from build123d import *

# Parameters (mm, degrees)
SKETCH1_W           = 6.5
SKETCH1_H           = 6
BOSS_EXTRUDE1_DEPTH = 1.75
SKETCH2_W           = 6.52
SKETCH2_H           = 6.02
SKETCH2_R           = 1.505
BOSS_EXTRUDE2_DEPTH = 0.25
SKETCH3_R           = 1.5
BOSS_EXTRUDE3_DEPTH = 1.2
FILLET1_R           = 0.1
SKETCH4_W           = 1.375
SKETCH4_H           = 0.75
BOSS_EXTRUDE4_DEPTH = 0.5


with BuildPart() as part:
    # Sketch1 → Boss-Extrude1 (new body)
    with BuildSketch(Plane(origin=(0, 0, 0), x_dir=(1, 0, 0), z_dir=(0, 1, 0))):
        Rectangle(SKETCH1_W, SKETCH1_H)
    extrude(amount=BOSS_EXTRUDE1_DEPTH)

    # Sketch2 → Boss-Extrude2 (add)
    with BuildSketch(Plane(origin=(0, 1.75, 0), x_dir=(1, 0, 0), z_dir=(0, 1, 0))):
        Rectangle(SKETCH2_W, SKETCH2_H)
        Circle(SKETCH2_R, mode=Mode.SUBTRACT)
    extrude(amount=BOSS_EXTRUDE2_DEPTH)

    # Sketch3 → Boss-Extrude3 (add)
    with BuildSketch(Plane(origin=(0, 1.75, 0), x_dir=(1, 0, 0), z_dir=(0, 1, 0))):
        Circle(SKETCH3_R)
    extrude(amount=BOSS_EXTRUDE3_DEPTH)

    # Fillet1
    fillet1_edges = [part.edges().sort_by_distance(p)[0] for p in [
        (-1.5, 2.95, 0),
    ]]
    fillet(fillet1_edges, radius=FILLET1_R)

    # Sketch4 → Boss-Extrude4 (add)
    with BuildSketch(Plane.XZ):
        with Locations((3.9375, 2.225)):
            Rectangle(SKETCH4_W, SKETCH4_H)
        with Locations((3.9375, -2.225)):
            Rectangle(SKETCH4_W, SKETCH4_H)
        with Locations((-3.9375, -2.225)):
            Rectangle(SKETCH4_W, SKETCH4_H)
        with Locations((-3.9375, 2.225)):
            Rectangle(SKETCH4_W, SKETCH4_H)
        with Locations((-3.9375, 0)):
            Rectangle(SKETCH4_W, SKETCH4_H)
    extrude(amount=-BOSS_EXTRUDE4_DEPTH)


solid = part.part
Here's how the part is built. I have some questions about the finished solid (model axes, mm). A direction names the side the tool comes from. Round coordinates to 2 decimals unless told otherwise and drop trailing zeros. Order: outer loops, then holes, each group sorted by start corner. A loop starts at its lowest first (then second) coordinate and runs counter-clockwise, first axis right, second up. Notation, with made-up numbers: M -15.5,-10 L 20.5,-10 A19 cw 20.5,1 Z; hole C 31,87.25 d10. An arc over 180 degrees is marked long. One line per question, with ' | ' between items.
1) Imagine slicing it at D-D, the plane y = 2.1. Write out the boundary of the cut face in (x, z), plus the area to 3 significant figures.
Checked values:
outline: C 0,0 d3 | area: 7.07 mm²
2) I'm going to push flat-ended pins straight in: pin 1 Ø0.6 at (x, y) = (-3.5, 0.5) entering from -Z; pin 2 Ø0.8 at (x, z) = (-4, 0) entering from +Y; pin 3 Ø0.6 at (x, y) = (-4, 0.5) entering from +Z. Where does each tip first touch, or does it pass through?
Checked values:
pin 1: stops at z = -3 | pin 2: stops at y = 0.5 | pin 3: stops at z = 2.6
3) Imagine slicing it at A-A, the plane x = 0. Write out the boundary of the cut face in (y, z) (3 decimals), plus the area to 3 significant figures.
Checked values:
outline: M 0,-3 L 1.75,-3 L 1.75,-3.01 L 2,-3.01 L 2,-1.505 L 1.75,-1.505 L 1.75,-1.5 L 2.85,-1.5 A0.1 ccw 2.95,-1.4 L 2.95,1.4 A0.1 ccw 2.85,1.5 L 1.75,1.5 L 1.75,1.505 L 2,1.505 L 2,3.01 L 1.75,3.01 L 1.75,3 L 0,3 Z | area: 14.8 mm²
4) On a 3-axis mill with a long thin cutter (end or side, diameter ignored), from which of +Z, -Z, +X, -X, +Y, -Y can I reach the whole of each face in a straight line? I mean faces 3 (the flat face through (0, 1, -3)), 4 (the flat face through (-1.5, 2, -0.7)), 5 (the flat face through (0, 2.95, 0)). Say none if no direction works.
Checked values:
face 3: -Z, +X, -X, -Y | face 4: +Y | face 5: +Z, -Z, +X, -X, +Y
5) I need wall thicknesses on line 1 (Y direction, x = 4, z = -2.5); line 2 (Z direction, x = -2.25, y = 0.1); line 3 (Y direction, x = -3, z = 1). Which ranges of each line are inside material? Lowest first, please.
Checked values:
line 1: y = 0 to 0.5 | line 2: z = -3 to 3 | line 3: y = 0 to 2
6) We'd pull the mould along X, two halves only. Please class faces 1 (the cylindrical face through (-1.5, 2.29, -0.07)), 2 (the flat face through (0, 1, 3)): released by +X, released by -X, zero draft, split by the parting line, or undercut.
Checked values:
face 1: undercut | face 2: zero draft
